Source: three-view drawing plus pictorial views. Frame: mm from the lowest corner of the part. A direction names the side the tool comes from. Give positions to 0.01 mm unless a question says otherwise; leave off trailing zeros. Write each loop counter-clockwise with the first axis right and the second up, starting at its lowest first coordinate (ties: lowest second). Pieces come first, ordered by that corner, then holes. Notation, with made-up numbers: (-21, 18.25) -> (2, 18.25) arc R15 ccw to (2, 29.25) -> close; hole circle Ø6 at (42.25, -35.5). An arc over 180 degrees is marked (long way). Use a Markdown table: item, result. Add a question column.
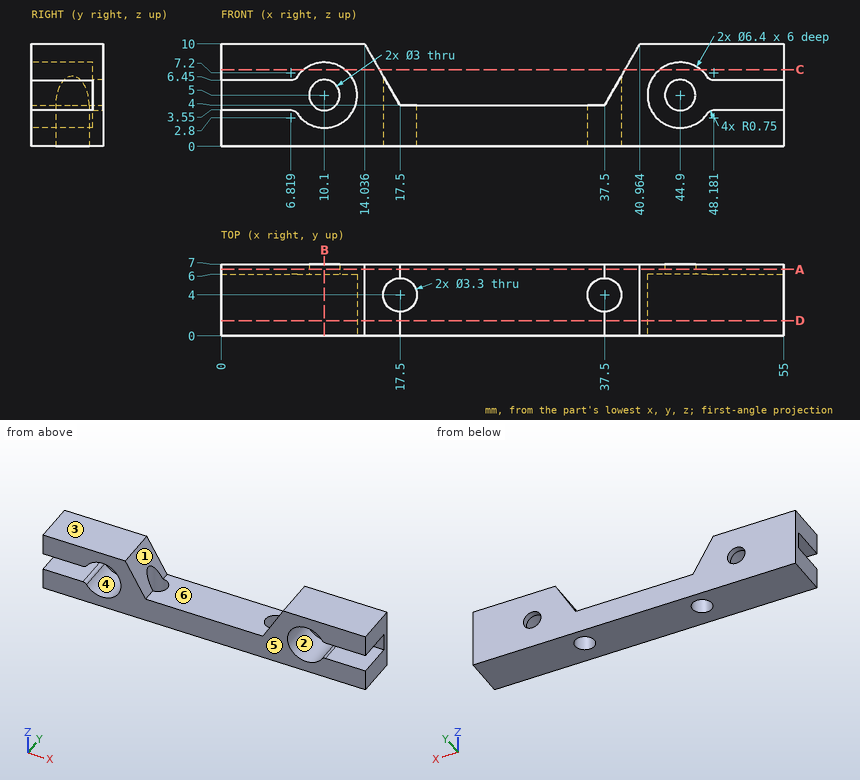
(1) Cut plane B-B on x = 10.1. Return the cut outline in (y, z), then the cut area to 3 significant figures.
(2) First-contact query: pin 1 Ø3.5 at (x, y) = (31.5, 3) entering from +Z; pin 2 Ø1.5 at (y, z) = (3, 5.5) entering from -X (1 decimal). Flat tips, straight axial feed; report the tip coordinate or a pass-through.
(3) Cut plane D-D on y = 1.5. Return the cut outline in (x, z).
(4) Access query for the marked faces 1, 2 and 3. Directions: +Z, -Z, +X, -X, +Y, -Y. A direction counts if a zero-diameter tool reaches every point of the face in a straight line with its end or side. Return the directions, or none.
(5) Material intervals for L1, parallel to X at y = 4, z = 1.5; L2, parallel to X at y = 6.2, z = 5; L3, parallel to Z at x = 10.1, y = 2.3, sorted ascending.
(6) Mould query, pull axis Z, two halves, no side actions, for the marked faces 4, 5 and 6. Classes: +Z half, -Z half, draft (parallel to the pull), parting line (faces both ways), or undercut.
(7) Cut plane A-A on y = 6.5. Return the cut outline in (x, z), then the cut area to 3 significant figures.
(8) Cut plane C-C on z = 7.5. Return the cut outline in (x, y).
Output:
| question | item | result |
|---|---|---|
| 1 | outline | (0, 0) -> (7, 0) -> (7, 3.5) -> (6, 3.5) -> (6, 1.8) -> (0, 1.8) -> close; (0, 8.2) -> (6, 8.2) -> (6, 6.5) -> (7, 6.5) -> (7, 10) -> (0, 10) -> close |
| 1 | area | 28.6 mm^2 |
| 2 | pin 1 | z = 4 |
| 2 | pin 2 | x = 13 |
| 3 | outline | (0, 0) -> (55, 0) -> (55, 3.55) -> (48.18, 3.55) arc R0.75 ccw to (47.56, 3.22) arc R3.2 cw (long way) to (47.56, 6.78) arc R0.75 ccw to (48.18, 6.45) -> (55, 6.45) -> (55, 10) -> (40.96, 10) -> (37.5, 4) -> (17.5, 4) -> (14.04, 10) -> (0, 10) -> (0, 6.45) -> (6.82, 6.45) arc R0.75 ccw to (7.44, 6.78) arc R3.2 cw (long way) to (7.44, 3.22) arc R0.75 ccw to (6.82, 3.55) -> (0, 3.55) -> close |
| 4 | face 1 | +Z, +Y, -Y |
| 4 | face 2 | -Y |
| 4 | face 3 | +Z, +X, -X, +Y, -Y |
| 5 | L1 | 0 to 15.85, 19.15 to 35.85, 39.15 to 55 |
| 5 | L2 | 0 to 8.6, 11.6 to 16.92, 38.08 to 43.4, 46.4 to 55 |
| 5 | L3 | 0 to 1.8, 8.2 to 10 |
| 6 | face 4 | undercut |
| 6 | face 5 | draft |
| 6 | face 6 | +Z half |
| 7 | outline | (0, 0) -> (55, 0) -> (55, 10) -> (40.96, 10) -> (37.5, 4) -> (17.5, 4) -> (14.04, 10) -> (0, 10) -> close; hole circle Ø3 at (10.1, 5); hole circle Ø3 at (44.9, 5) |
| 7 | area | 395 mm^2 |
| 8 | outline | (0, 0) -> (8.1, 0) -> (8.1, 6) -> (12.1, 6) -> (12.1, 0) -> (15.48, 0) -> (15.48, 7) -> (0, 7) -> close; (39.52, 0) -> (42.9, 0) -> (42.9, 6) -> (46.9, 6) -> (46.9, 0) -> (55, 0) -> (55, 7) -> (39.52, 7) -> close |
